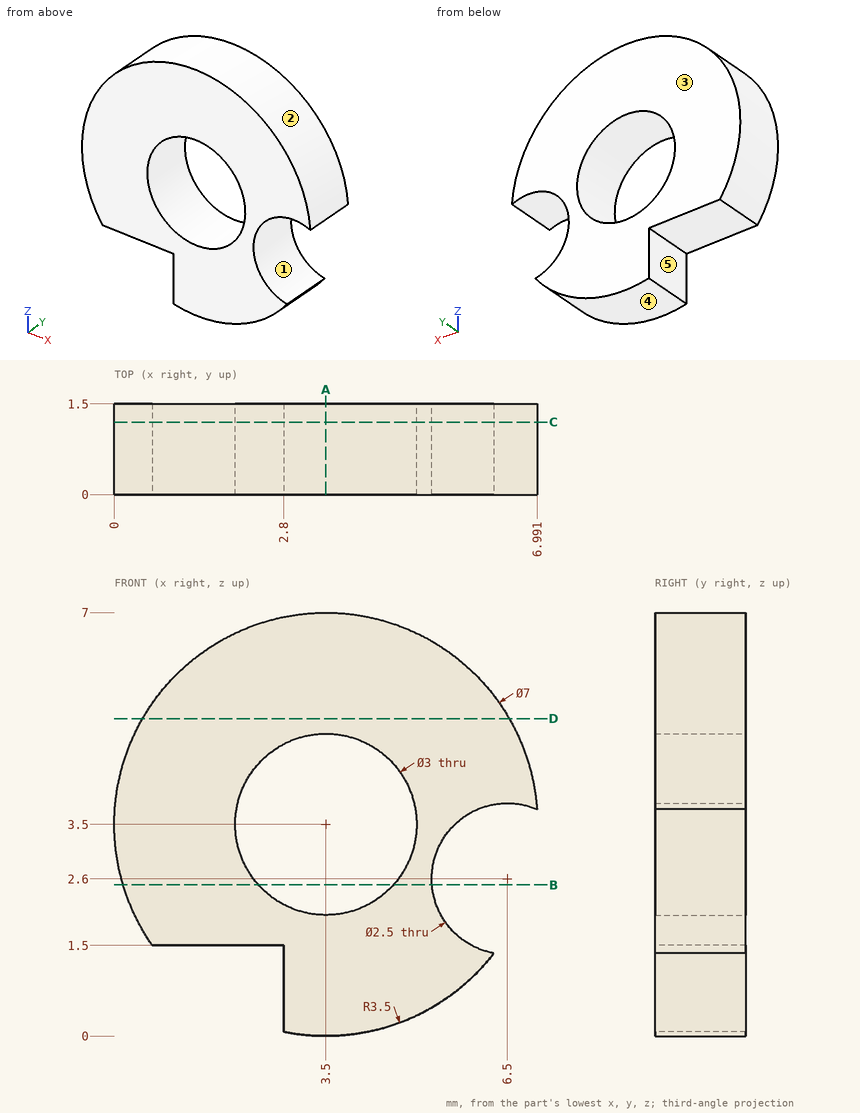
Drawing for the job (mm, zero at the part's lowest x, y, z). A direction names the side the tool comes from. Round coordinates to 2 decimals unless told otherwise and drop trailing zeros. Order: outer loops, then holes, each group sorted by start corner. A loop starts at its lowest first (then second) coordinate and runs counter-clockwise, first axis right, second up. Notation, with made-up numbers: (79.25, -4.5) -> (106.25, -4.5) arc R22 cw to (106.25, 16.5) -> close; hole circle Ø2 at (37, 54.25). An arc over 180 degrees is marked (long way). Put each result on its own line as item: value.
Q1. Band-saw the part on A-A (x = 3.5). Give the cut face in (y, z), and give its area (3 significant figures).
From the geometry:
outline: (0, 0) -> (1.5, 0) -> (1.5, 2) -> (0, 2) -> close; (0, 5) -> (1.5, 5) -> (1.5, 7) -> (0, 7) -> close
area: 6.00 mm2
Q2. Tool access for the marked faces 4 and 5: list every direction of +Z, -Z, +X, -X, +Y, -Y with a clear straight run to the whole face (end or side of a thin tool).
From the geometry:
face 4: -Z, +Y, -Y
face 5: -Z, -X, +Y, -Y
Q3. Band-saw the part on D-D (z = 5.25). Give the cut face in (x, y).
From the geometry:
outline: (0.47, 0) -> (6.53, 0) -> (6.53, 1.5) -> (0.47, 1.5) -> close
Q4. Band-saw the part on C-C (y = 1.2). Give the cut face in (x, z), and give its area (3 significant figures).
From the geometry:
outline: (0.63, 1.5) -> (2.8, 1.5) -> (2.8, 0.07) arc R3.5 ccw to (6.28, 1.37) arc R1.25 cw (long way) to (6.99, 3.75) arc R3.5 ccw (long way) to start; hole circle Ø3 at (3.5, 3.5)
area: 26.2 mm2
Q5. Wall check: line 1 (X direction, y = 0.8, z = 2.25); line 2 (X direction, y = 0.3, z = 2.75); line 3 (Z direction, x = 5.5, y = 0.8). Give the ranges that are in metal, low to high. Write a range as [from, to].
From the geometry:
line 1: x = [0.23, 2.67], [4.33, 5.3]
line 2: x = [0.08, 2.2], [4.8, 5.26]
line 3: z = [0.63, 1.85], [3.35, 6.37]
Q6. Pull direction X, two halves, no side cores. Call the marked faces 1, 2 and 3: pulls with the +X half, pulls with the -X half, needs draft (parallel to the pull), parting line crosses it, or undercut.
From the geometry:
face 1: undercut
face 2: parting line crosses it
face 3: needs draft
Q7. Band-saw the part on B-B (z = 2.5). Give the cut face in (x, y), and give its area (3 significant figures).
From the geometry:
outline: (0.15, 0) -> (2.38, 0) -> (2.38, 1.5) -> (0.15, 1.5) -> close; (4.62, 0) -> (5.25, 0) -> (5.25, 1.5) -> (4.62, 1.5) -> close
area: 4.31 mm2
